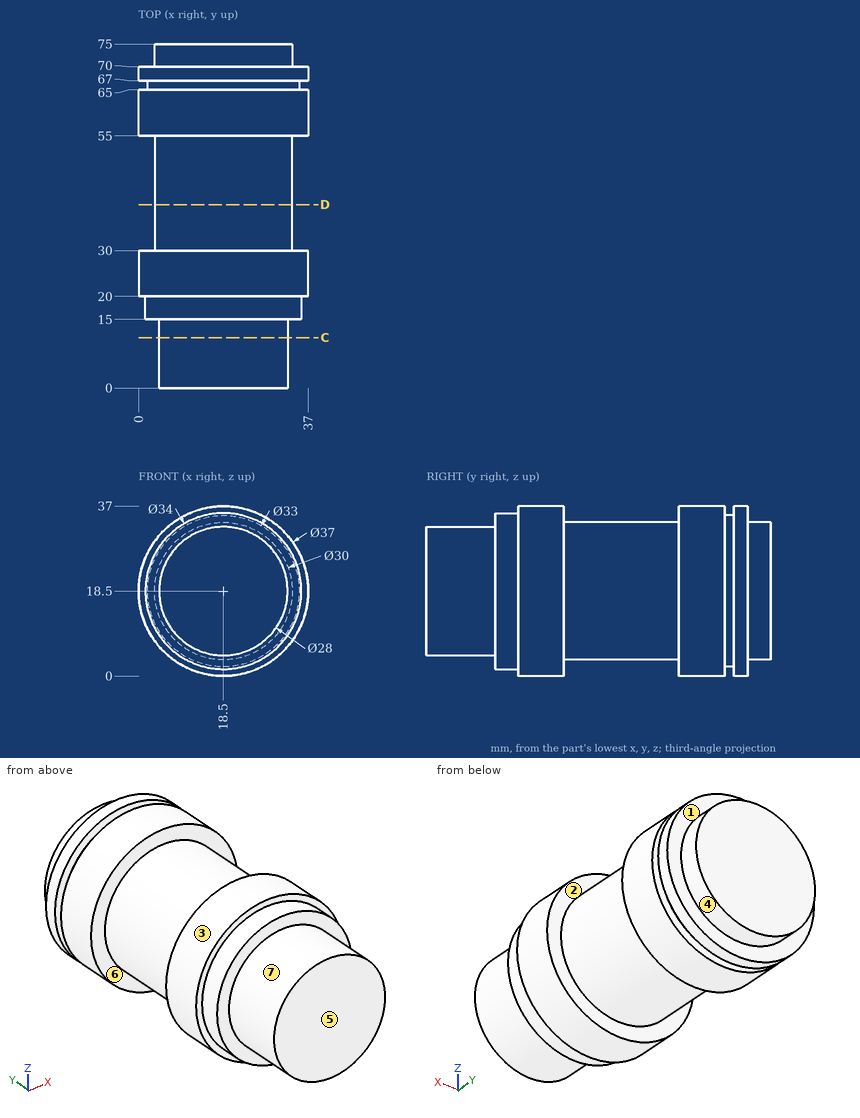
For this review, use the dimensioned drawing (mm, ordinates from the lowest corner) and the shaded views. A direction names the side the tool comes from. Coordinates: 2 decimals unless noted, no trailing zeros. Loops run counter-clockwise (first coordinate to the right, second up) from the corner with the lowest first, then second, coordinate; pieces in that order, holes last. Notation, with made-up numbers: M 75,-37.75 L 84,-37.75 A30 ccw 84,-5.75 Z; hole C 71.5,5 d3. An arc over 180 degrees is marked long. Answer as CSV lines item,"result".
Item 1: Add section C-C on y = 11. State the section outline as (x, z) points.
Answer list:
outline,"C 18.5,18.5 d28"
Item 2: Add section D-D on y = 40. State the section outline as (x, z) points, plus the area to 3 significant figures.
Answer list:
outline,"C 18.5,18.5 d30"
area,"707 mm²"
Item 3: Machinability: for the marked faces 4, 5, 6 and 7, which of the approach directions +Z, -Z, +X, -X, +Y, -Y give a long, thin tool a straight path to every point of the face, cutting with its end or side? Answer none if there is none.
Answer list:
face 4,"+Y"
face 5,"+Z, -Z, +X, -X, -Y"
face 6,"none"
face 7,"-Y"
Item 4: For P1, Ø2, axis at y = 42.5, z = 7, coming from the -X side; P2, Ø5, axis at x = 3.5, z = 27, coming from the -Y side; P3, Ø10, axis at x = 26.5, y = 16, coming from the -Z side, all flat-tipped, find the tip position at first contact; note any pin that passes through.
Answer list:
P1,"x = 7.79"
P2,"y = 15"
P3,"z = 0.69"
Item 5: For probe 1 along Y at (x, z) = (28, 6.5); probe 2 along Y at (x, z) = (4.5, 17); probe 3 along X at (y, z) = (70.5, 18), list the stretches that pass through material, from the lowest coordinate up.
Answer list:
probe 1,"15 to 30, 55 to 70"
probe 2,"15 to 75"
probe 3,"3.51 to 33.49"
Item 6: The part is to be moulded in two halves that separate along Y. For the marked faces 1, 2 and 3, say which applies: pulls with the +Y half, pulls with the -Y half, needs draft (parallel to the pull), parting line crosses it, or undercut.
Answer list:
face 1,"pulls with the +Y half"
face 2,"undercut"
face 3,"needs draft"
